from build123d import *

# Parameters (mm, degrees)
SKETCH3_R           = 27.7
BOSS_EXTRUDE2_DEPTH = 11
SKETCH4_R           = 30
BOSS_EXTRUDE3_DEPTH = 2
SKETCH5_R           = 2.2
CUT_EXTRUDE1_DEPTH  = 44.829214002


with BuildPart() as part:
    # Sketch3 → Boss-Extrude2 (new body)
    with BuildSketch(Plane(origin=(0, 0, 0), x_dir=(1, 0, 0), z_dir=(0, 1, 0))):
        with Locations(Location((0, 0, 0), (0, 0, 270))):
            Circle(SKETCH3_R)
    extrude(amount=BOSS_EXTRUDE2_DEPTH)

    # Sketch4 → Boss-Extrude3 (add)
    with BuildSketch(Plane(origin=(0, 0, 0), x_dir=(1, 0, 0), z_dir=(0, 1, 0))):
        with Locations(Location((0, 0, 0), (0, 0, 270))):
            Circle(SKETCH4_R)
    extrude(amount=BOSS_EXTRUDE3_DEPTH)

    # Sketch5 → Cut-Extrude1 (cut, through all)
    with BuildSketch(Plane(origin=(0, 11, 0), x_dir=(1, 0, 0), z_dir=(0, 1, 0))):
        with Locations(Location((0, 24, 0), (0, 0, 270))):
            Circle(SKETCH5_R)
        with Locations(Location((22.825356391, 7.416407865, 0), (0, 0, 270))):
            Circle(SKETCH5_R)
        with Locations(Location((14.106846055, -19.416407865, 0), (0, 0, 270))):
            Circle(SKETCH5_R)
        with Locations(Location((-14.106846055, -19.416407865, 0), (0, 0, 270))):
            Circle(SKETCH5_R)
        with Locations(Location((-22.825356391, 7.416407865, 0), (0, 0, 270))):
            Circle(SKETCH5_R)
    extrude(amount=-CUT_EXTRUDE1_DEPTH, mode=Mode.SUBTRACT)


solid = part.part
Here's how the part is built. I have some questions about the finished solid (model axes, mm). A direction names the side the tool comes from. Coordinates: 2 decimals unless noted, no trailing zeros. Order: outer loops, then holes, each group sorted by start corner. A loop starts at its lowest first (then second) coordinate and runs counter-clockwise, first axis right, second up.
Item 1: If we section it at B-B on z = 19: List the corners of the cut face in (x, y) for me, plus the area to 3 significant figures.
Result sheet:
outline: (-23.22, 0) - (-16.27, 0) - (-16.27, 11) - (-20.16, 11) - (-20.16, 2) - (-23.22, 2) - close; (-11.95, 0) - (11.95, 0) - (11.95, 11) - (-11.95, 11) - close; (16.27, 0) - (23.22, 0) - (23.22, 2) - (20.16, 2) - (20.16, 11) - (16.27, 11) - close
area: 361 mm2
Item 2: If we section it at A-A on x = 0: List the corners of the cut face in (y, z) for me, plus the area to 3 significant figures.
Result sheet:
outline: (0, -30) - (2, -30) - (2, -27.7) - (11, -27.7) - (11, -26.2) - (0, -26.2) - close; (0, -21.8) - (11, -21.8) - (11, 27.7) - (2, 27.7) - (2, 30) - (0, 30) - close
area: 570 mm2
Item 3: I need wall thicknesses on line 1 (X direction, y = 6, z = 20); line 2 (Z direction, x = -14, y = 8.25); line 3 (Z direction, x = -23.5, y = 6.5). Which ranges of each line are inside material? Lowest first, please.
Result sheet:
line 1: x = -19.16 to -16.23, -11.99 to 11.99, 16.23 to 19.16
line 2: z = -23.9 to 17.22, 21.61 to 23.9
line 3: z = -14.66 to -9.51, -5.32 to 14.66
Item 4: If we section it at C-C on z = -25.5: List the corners of the cut face in (x, y) for me.
Result sheet:
outline: (-15.8, 0) - (-1.61, 0) - (-1.61, 11) - (-10.82, 11) - (-10.82, 2) - (-15.8, 2) - close; (1.61, 0) - (15.8, 0) - (15.8, 2) - (10.82, 2) - (10.82, 11) - (1.61, 11) - close
Item 5: For faces 4 (the face through (-11.926, 5.577, 19.13)), 5 (the face through (-27.041, 6.437, -6.005)), which set-ups out of +Z, -Z, +X, -X, +Y, -Y let a thin tool reach every point of the face, with its end or its side?
Result sheet:
face 4: +Y, -Y
face 5: +Y
Item 6: If we section it at D-D on y = 8.5: List the corners of the cut face in (x, z) for me.
Result sheet:
outline: circle Ø55.4 at (0, 0); hole circle Ø4.4 at (-22.83, -7.42); hole circle Ø4.4 at (-14.11, 19.42); hole circle Ø4.4 at (0, -24); hole circle Ø4.4 at (14.11, 19.42); hole circle Ø4.4 at (22.83, -7.42)
Item 7: For P1, Ø5, axis at y = 2.5, z = -17, coming from the +X side; P2, Ø6, axis at x = -4, y = 7.5, coming from the +Z side; P3, Ø2, axis at x = -12, y = 4, coming from the +Z side, each with a flat end and sliding along its axis, tell me the tip position at first contact or that it passes through.
Result sheet:
P1: stops at x = 26.24
P2: stops at z = 27.68
P3: stops at z = 25.42
Item 8: If we mould it in two halves opening along X, with no side actions, what happens to faces 1 (the face through (1.32, 0.99, -29.97)), 2 (the face through (-27, 2, 9)), 3 (the face through (-21.3, 5.6, -9))? For each: +X half, -X half, draft (parallel to the pull), parting line (faces both ways), or undercut.
Result sheet:
face 1: parting line
face 2: draft
face 3: undercut
